Work out the finished part from the listing and answer in its coordinate system (mm). A direction names the side the tool comes from. Round coordinates to 2 decimals unless told otherwise and drop trailing zeros. Order: outer loops, then holes, each group sorted by start corner. A loop starts at its lowest first (then second) coordinate and runs counter-clockwise, first axis right, second up. Notation, with made-up numbers: (82, -23) - (135, -23) arc R31 cw to (135, 3) - close; hole circle Ø9 at (-2.5, 14.5). An arc over 180 degrees is marked (long way). Use one line per item in the form item = value. Start each with the question number.
Q1. Find the intervals of material crossed by line 1 (Y direction, x = -9, z = 9.5); line 2 (X direction, y = 212.5, z = 12.5); line 3 (Y direction, x = 2.5, z = -14), in increasing order. Write a range as [from, to].
Q2. For a pull along X with two mould halves and no side action, classify faces 1 (the flat face through (8, 221.5, 0)), 2 (the flat face through (-4, 216, 0)), 3 (the cylindrical face through (6.13, 210.87, 14.78)), 4 (the flat face through (0, 211.5, 0)) as +X half, -X half, draft (parallel to the pull), parting line (faces both ways), or undercut.
Q3. Given P1, Ø1, axis at x = 1, z = -0.5, coming from the +Y side; P2, Ø12, axis at y = 50.5, z = -12, coming from the -X side; P3, Ø3, axis at x = -3, y = 100, coming from the -Z side, each flat-ended and moving along its own axis, determine where each tip first touches the part or whether it passes through.
Q4. Which of the six approach directions +Z, -Z, +X, -X, +Y, -Y give full straight-line access (tool end or side, diameter ignored) to faces 5 (the conical face through (-15.16, 221.34, 0.28)), 6 (the flat face through (7, 201.5, 7)), 7 (the flat face through (4, 216, 0))?
Q5. The part is cut by section A-A on y = 151. Determine the outline of the cut face in (x, z).
from build123d import *

# Parameters (mm, degrees)
CHAMFER_1_SIZE           = 9
CUT_EXTRUDE_1_DEPTH      = 223.652756552
CUT_EXTRUDE_1_DEPTH_BACK = 223.652756552
SKETCH_2_W               = 8
SKETCH_2_H               = 10
CHAMFER_2_SIZE           = 1


with BuildPart() as part:
    # Эскиз1 → Повернуть1 (revolve)
    with BuildSketch(Plane.XY, mode=Mode.PRIVATE) as revolve_1_sk:
        Polygon((0, 0), (0, 221.5), (16, 221.5), (16, 201.5), (9, 201.5), (9, 0), align=None)
    revolve(revolve_1_sk.sketch.rotate(Axis((0, 0, 0), (0, -1, 0)), 90), axis=Axis((0, 0, 0), (0, -1, 0)))

    # Фаска1
    chamfer_1_edges = [part.edges().sort_by_distance(p)[0] for p in [
        (0, 0, -9),
    ]]
    chamfer(chamfer_1_edges, length=CHAMFER_1_SIZE - 0.0001)  # a hair under: the kernel refuses the full size

    # Эскиз2 → Вырез-Вытянуть1 (cut, two sides: drawn at the far end of the back side and taken through both)
    with BuildSketch(Plane.XY.offset(-CUT_EXTRUDE_1_DEPTH_BACK)):
        with Locations((0, 216.5)):
            Rectangle(SKETCH_2_W, SKETCH_2_H)
    extrude(amount=CUT_EXTRUDE_1_DEPTH + CUT_EXTRUDE_1_DEPTH_BACK, mode=Mode.SUBTRACT)

    # Фаска2
    chamfer_2_edges = [part.edges().sort_by_distance(p)[0] for p in [
        (16, 221.5, 0),
        (-16, 221.5, 0),
    ]]
    chamfer(chamfer_2_edges, length=CHAMFER_2_SIZE)


solid = part.part
Found:
q1.line_1 = [201.5, 221.5]
q1.line_2 = [-9.99, -4], [4, 9.99]
q1.line_3 = [201.5, 211.5]
q2.face_1 = draft
q2.face_2 = undercut
q2.face_3 = parting line
q2.face_4 = undercut
q3.P1 = 211.5
q3.P2 = -6.71
q3.P3 = -8.87
q4.face_5 = -X, +Y
q4.face_6 = -Y
q4.face_7 = +Z, -Z, +Y
q5.outline = circle Ø18 at (0, 0)
